from build123d import *

# Parameters (mm, degrees)
F0_W   = 0.76
F0_H   = 4.215
F0_W_2 = 12.7
F0_H_2 = 2.85


with BuildPart() as f1:
    # F0 (on Right) → F1 (revolve)
    with BuildSketch(Plane.YZ):
        Polygon((0, 4.35), (0, 0), (0.45, 0), (1.14, 0), (1.14, 4.215), (1.14, 4.8), (0.45, 4.8), align=None)
        with Locations((1.52, 2.1075)):
            Rectangle(F0_W, F0_H)
        Polygon((1.9, 4.215), (1.9, 0), (3.13, 0), (3.13, 4.79), align=None)
        Polygon((3.13, 4.79), (3.13, 0), (36.52, 0), (36.52, 4.5), align=None)
        Polygon((36.52, 4.5), (36.52, 0), (39.55, 0), (44.7, 0), (44.7, 2.85), (44.7, 3.215), (39.55, 3.215), align=None)
        with Locations((51.05, 1.425)):
            Rectangle(F0_W_2, F0_H_2)
    revolve(axis=Axis((0, 19.825, 0), (0, 1, 0)))


solid = f1.part
The model under review builds one solid part; all positions refer to its coordinate system, in mm. A direction names the side the tool comes from. Coordinates: 2 decimals unless noted, no trailing zeros. Write each loop counter-clockwise with the first axis right and the second up, starting at its lowest first coordinate (ties: lowest second). Pieces come first, ordered by that corner, then holes. Notation, with made-up numbers: (36, 78) - (59, 78) arc R7 ccw to (59, 83) - close; hole circle Ø7 at (74.5, 54). An arc over 180 degrees is marked (long way). Answer as a JSON object with one key per item and string values. Group by question number.
1. Machinability: for faces 5 (the face through (4.05, 0.79, 2.58)), 6 (the face through (-1.96, 42.09, -2.55)), 7 (the face through (-4.115, 1.525, -0.914)), which of the approach directions +Z, -Z, +X, -X, +Y, -Y give a long, thin tool a straight path to every point of the face, cutting with its end or side? Answer none if there is none.
2. Add section B-B (y = 38.5). Give the boundary of the cut face in (x, z), plus the area to 3 significant figures.
3. Mouldability with a two-part tool opening along Y and no side actions: class faces 1 (the face through (-1.734, 51.139, -2.262)), 2 (the face through (-4, 1.14, -2)), 3 (the face through (3.267, 39.36, -0.429)), 4 (the face through (0, 0, 0)) as pulls with the +Y half, pulls with the -Y half, needs draft (parallel to the pull), parting line crosses it, or undercut.
4. Clearance check with flat-ended pins moving along their axes: pin 1 Ø4 at (x, z) = (-1, -1) entering from -Y; pin 2 Ø1 at (x, y) = (0.5, 34) entering from -Z; pin 3 Ø4 at (x, y) = (0.5, 34.5) entering from +Z; pin 4 Ø2 at (y, z) = (27, 3.5) entering from -X. State where each tip first meets the part, or that it passes through.
5. To check wall thickness, follow probe 1 along X at (y, z) = (29.5, -0.75); probe 2 along Y at (x, z) = (3, -3.25); probe 3 along Y at (x, z) = (-3.5, -2.5). State the ranges of each line that lie inside material, in increasing order.
6. Add section A-A (y = 50.5). Give the boundary of the cut face in (x, z), plus the area to 3 significant figures.
Findings:
{
 "1": {"face 5": "+Y, -Y", "face 6": "+Y", "face 7": "none"},
 "2": {"outline": "circle Ø7.32 at (0, 0)", "area": "42.1 mm²"},
 "3": {"face 1": "needs draft", "face 2": "undercut", "face 3": "pulls with the +Y half", "face 4": "pulls with the -Y half"},
 "4": {"pin 1": "y = 0", "pin 2": "z = -4.52", "pin 3": "z = 4.53", "pin 4": "x = -3.84"},
 "5": {"probe 1": "-4.5 to 4.5", "probe 2": "0.07 to 1.14, 2.34 to 36.7", "probe 3": "0 to 1.14, 2.08 to 36.99"},
 "6": {"outline": "circle Ø5.7 at (0, 0)", "area": "25.5 mm²"}
}
